from build123d import *

# Parameters (mm, degrees)
ESQUISSE1_W             = 38
ESQUISSE1_H             = 24
BOSS_EXTRU_1_DEPTH      = 20
ESQUISSE2_W             = 32
ESQUISSE2_H             = 18
ENL_V_MAT_EXTRU_1_DEPTH = 12
ESQUISSE3_W             = 30
ESQUISSE3_H             = 5
ENL_V_MAT_EXTRU_2_DEPTH = 30
ESQUISSE4_W             = 20
ESQUISSE4_H             = 5
ENL_V_MAT_EXTRU_3_DEPTH = 60
ESQUISSE5_R             = 2.5
ENL_V_MAT_EXTRU_4_DEPTH = 60


with BuildPart() as part:
    # Esquisse1 → Boss.-Extru.1 (new body)
    with BuildSketch(Plane(origin=(0, 0, 0), x_dir=(1, 0, 0), z_dir=(0, 1, 0))):
        Rectangle(ESQUISSE1_W, ESQUISSE1_H)
    extrude(amount=BOSS_EXTRU_1_DEPTH)

    # Esquisse2 → Enlèv. mat.-Extru.1 (cut)
    with BuildSketch(Plane(origin=(0, 20, 0), x_dir=(1, 0, 0), z_dir=(0, 1, 0))):
        Rectangle(ESQUISSE2_W, ESQUISSE2_H)
    extrude(amount=-ENL_V_MAT_EXTRU_1_DEPTH, mode=Mode.SUBTRACT)

    # Esquisse3 → Enlèv. mat.-Extru.2 (cut)
    with BuildSketch(Plane.XY.offset(12)):
        with Locations((0, 1.5)):
            Rectangle(ESQUISSE3_W, ESQUISSE3_H)
    extrude(amount=-ENL_V_MAT_EXTRU_2_DEPTH, mode=Mode.SUBTRACT)

    # Esquisse4 → Enlèv. mat.-Extru.3 (cut)
    with BuildSketch(Plane.ZY.offset(19)):
        with Locations((0, 1.5)):
            Rectangle(ESQUISSE4_W, ESQUISSE4_H)
    extrude(amount=-ENL_V_MAT_EXTRU_3_DEPTH, mode=Mode.SUBTRACT)

    # Esquisse5 → Enlèv. mat.-Extru.4 (cut)
    with BuildSketch(Plane(origin=(0, 8, 0), x_dir=(1, 0, 0), z_dir=(0, 1, 0))):
        with Locations(Location((0, 0, 0), (0, 0, 270))):
            Circle(ESQUISSE5_R)
    extrude(amount=-ENL_V_MAT_EXTRU_4_DEPTH, mode=Mode.SUBTRACT)


solid = part.part
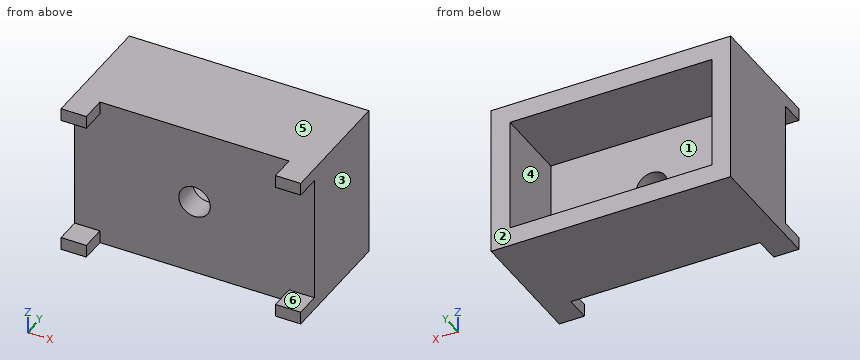
For this review, take the finished solid that the model builds, in its own axes (mm). Face numbers are marked on the shaded views. A direction names the side the tool comes from. Coordinates: 2 decimals unless noted, no trailing zeros. Order: outer loops, then holes, each group sorted by start corner. A loop starts at its lowest first (then second) coordinate and runs counter-clockwise, first axis right, second up. Notation, with made-up numbers: (18, 82) - (23, 82) arc R13 ccw to (23, 100) - close; hole circle Ø5 at (77, 19). An arc over 180 degrees is marked (long way). Use one line per item in the form item = value.
Q1. Consider section D-D (z = 6.5). Give the boundary of the cut face in (x, y).
Checked values:
outline = (-19, 4) - (19, 4) - (19, 20) - (16, 20) - (16, 8) - (-16, 8) - (-16, 20) - (-19, 20) - close
Q2. For probe 1 along Z at (x, y) = (-13, 17.5); probe 2 along X at (y, z) = (5.1, 0); probe 3 along X at (y, z) = (13.5, -8), list the stretches that pass through material, from the lowest coordinate up. Write a range as from..to.
Checked values:
probe_1 = -12..-9, 9..12
probe_2 = -19..-2.5, 2.5..19
probe_3 = -19..-16, 16..19
Q3. Consider section C-C (y = 13.5). Give the boundary of the cut face in (x, z), then the cut area to 3 significant figures.
Checked values:
outline = (-19, -12) - (19, -12) - (19, 12) - (-19, 12) - close; hole (-16, -9) - (16, -9) - (16, 9) - (-16, 9) - close
area = 336 mm2
Q4. For P1, Ø7, axis at x = -8.5, z = 0.5, coming from the -Y side; P2, Ø6, axis at x = 0, z = 0, coming from the +Y side, all flat-tipped, find the tip position at first contact; note any pin that passes through.
Checked values:
P1 = 4
P2 = 8
Q5. Consider section A-A (x = 0). Give the boundary of the cut face in (y, z).
Checked values:
outline = (4, -12) - (20, -12) - (20, -9) - (8, -9) - (8, -2.5) - (4, -2.5) - close; (4, 2.5) - (8, 2.5) - (8, 9) - (20, 9) - (20, 12) - (4, 12) - close
Q6. For the marked faces 4, 5 and 6, list the 3-axis set-ups (+Z, -Z, +X, -X, +Y, -Y) from which the entire face can be reached by the end or side of a thin tool; tool diameter is ignored.
Checked values:
face_4 = +Y
face_5 = +Z, +X, -X, +Y, -Y
face_6 = +X, -X, -Y
Q7. Draft analysis for pull direction X (two halves, no side actions). For the marked faces 1, 2 and 3, state which applies: +X half, -X half, draft (parallel to the pull), parting line (faces both ways), or undercut.
Checked values:
face_1 = undercut
face_2 = draft
face_3 = +X half
Q8. Consider section B-B (z = 0). Give the boundary of the cut face in (x, y).
Checked values:
outline = (-19, 4) - (-2.5, 4) - (-2.5, 8) - (-16, 8) - (-16, 20) - (-19, 20) - close; (2.5, 4) - (19, 4) - (19, 20) - (16, 20) - (16, 8) - (2.5, 8) - close
